Autodesk Fusion 360 part; units mm, degrees
sketch "Sketch1" plane through (0, 0, 0) normal (0, 0, 1) x (1, 0, 0)
  line L0 (0, 0) -> (53.2, 0)
  line L1 (53.2, 0) -> (53.2, 40.2)
  line L2 (53.2, 40.2) -> (0, 40.2)
  line L3 (0, 40.2) -> (0, 0)
  circle A0 centre (4.6, 4.6) radius 1.75
  circle A1 centre (4.6, 35.6) radius 1.75
  circle A2 centre (48.6, 35.6) radius 1.75
  circle A3 centre (48.6, 4.6) radius 1.75
  dimension "d1" = 53.2
  dimension "d2" = 40.2
  dimension "d3" = 4.6
  dimension "d4" = 4.6
  dimension "d5" = 4.6
  dimension "d6" = 4.6
  dimension "d7" = 4.6
  dimension "d8" = 4.6
  dimension "d9" = 4.6
  dimension "d10" = 4.6
  dimension "d11" = 3.5
  dimension "d12" = 3.5
  dimension "d13" = 3.5
  dimension "d14" = 3.5
extrude "Extrude1" add sketch "Sketch1" along normal blind 4
fillet "Fillet1" radius 4.6 4 edges at (0, 40.2, 2) (0, 0, 2) (53.2, 0, 2) (53.2, 40.2, 2)
sketch "Sketch2" plane through (0, 0, 0) normal (0, 0, -1) x (-1, 0, 0)
  arc A0 (-48.6, 40.2) -> (-53.2, 35.6) centre (-48.6, 35.6) ccw
  line L0 (-53.2, 35.6) -> (-53.2, 4.6)
  arc A1 (-53.2, 4.6) -> (-48.6, 0) centre (-48.6, 4.6) ccw
  line L1 (-48.6, 0) -> (-4.6, 0)
  arc A2 (-4.6, 0) -> (0, 4.6) centre (-4.6, 4.6) ccw
  line L2 (0, 4.6) -> (0, 35.6)
  arc A3 (0, 35.6) -> (-4.6, 40.2) centre (-4.6, 35.6) ccw
  line L3 (-4.6, 40.2) -> (-48.6, 40.2)
  circle A4 centre (-48.6, 4.6) radius 1.75
  circle A5 centre (-48.6, 35.6) radius 1.75
  circle A6 centre (-4.6, 4.6) radius 1.75
  circle A7 centre (-4.6, 35.6) radius 1.75
  line L4 (-51.6, 35.6) -> (-51.6, 4.6)
  arc A8 (-51.6, 4.6) -> (-48.6, 1.6) centre (-48.6, 4.6) ccw
  line L5 (-48.6, 1.6) -> (-4.6, 1.6)
  arc A9 (-4.6, 1.6) -> (-1.6, 4.6) centre (-4.6, 4.6) ccw
  line L6 (-1.6, 4.6) -> (-1.6, 35.6)
  arc A10 (-1.6, 35.6) -> (-4.6, 38.6) centre (-4.6, 35.6) ccw
  line L7 (-4.6, 38.6) -> (-48.6, 38.6)
  arc A11 (-48.6, 38.6) -> (-51.6, 35.6) centre (-48.6, 35.6) ccw
  dimension "d18" = 1.6
extrude "Extrude2" cut sketch "Sketch2" against normal blind 2 contours L4 A8 L5 A9 L6 A10 L7 A11
sketch "Sketch3" plane through (0, 0, 0) normal (0, 0, -1) x (-1, 0, 0)
  line L0 (-51.6, 4.6) -> (-51.6, 35.6)
  arc A0 (-48.6, 38.6) -> (-51.6, 35.6) centre (-48.6, 35.6) ccw
  line L1 (-48.6, 38.6) -> (-4.6, 38.6)
  arc A1 (-1.6, 35.6) -> (-4.6, 38.6) centre (-4.6, 35.6) ccw
  line L2 (-1.6, 35.6) -> (-1.6, 4.6)
  arc A2 (-4.6, 1.6) -> (-1.6, 4.6) centre (-4.6, 4.6) ccw
  line L3 (-4.6, 1.6) -> (-48.6, 1.6)
  arc A3 (-51.6, 4.6) -> (-48.6, 1.6) centre (-48.6, 4.6) ccw
  arc A4 (-48.6, 40.2) -> (-53.2, 35.6) centre (-48.6, 35.6) ccw
  line L4 (-53.2, 35.6) -> (-53.2, 4.6)
  arc A5 (-53.2, 4.6) -> (-48.6, 0) centre (-48.6, 4.6) ccw
  line L5 (-48.6, 0) -> (-4.6, 0)
  arc A6 (-4.6, 0) -> (0, 4.6) centre (-4.6, 4.6) ccw
  line L6 (0, 4.6) -> (0, 35.6)
  arc A7 (0, 35.6) -> (-4.6, 40.2) centre (-4.6, 35.6) ccw
  line L7 (-4.6, 40.2) -> (-48.6, 40.2)
  line L8 (0, 24.6) -> (-1.6, 24.6)
  line L9 (0, 7.6) -> (-1.6, 7.6)
  line L10 (-53.2, 28.6) -> (-51.6, 28.6)
  line L11 (-53.2, 6.6) -> (-51.6, 6.6)
  line L12 (-46.35, 40.2) -> (-46.35, 38.6)
  line L13 (-7.35, 40.2) -> (-7.35, 38.6)
  dimension "d21" = 17
  dimension "d22" = 11
  dimension "d25" = 5
  dimension "d26" = 10
  dimension "d27" = 5.75
  dimension "d73" = 39
extrude "Extrude3" cut sketch "Sketch3" against normal blind 2 contours L0 L4 L10 L11 | L2 L6 L8 L9 | L1 L7 L12 L13
sketch "Sketch4" plane through (0, 0, 2) normal (0, 0, -1) x (-1, 0, 0)
  circle A0 centre (-48.6, 4.6) radius 1.75
  circle A1 centre (-4.6, 35.6) radius 1.75
  circle A2 centre (-4.6, 4.6) radius 1.75
  circle A3 centre (-48.6, 35.6) radius 1.75
  line L0 (-53.2, 28.6) -> (-53.2, 6.6)
  line L1 (0, 7.6) -> (0, 24.6)
  line L2 (-7.35, 40.2) -> (-46.35, 40.2)
  arc A4 (-48.6, 38.6) -> (-51.6, 35.6) centre (-48.6, 35.6) ccw
  line L3 (-51.6, 35.6) -> (-51.6, 28.6)
  line L4 (-51.6, 28.6) -> (-53.2, 28.6)
  line L5 (-53.2, 6.6) -> (-51.6, 6.6)
  line L6 (-51.6, 6.6) -> (-51.6, 4.6)
  arc A5 (-51.6, 4.6) -> (-48.6, 1.6) centre (-48.6, 4.6) ccw
  line L7 (-48.6, 1.6) -> (-4.6, 1.6)
  arc A6 (-4.6, 1.6) -> (-1.6, 4.6) centre (-4.6, 4.6) ccw
  line L8 (-1.6, 4.6) -> (-1.6, 7.6)
  line L9 (-1.6, 7.6) -> (0, 7.6)
  line L10 (0, 24.6) -> (-1.6, 24.6)
  line L11 (-1.6, 24.6) -> (-1.6, 35.6)
  arc A7 (-1.6, 35.6) -> (-4.6, 38.6) centre (-4.6, 35.6) ccw
  line L12 (-4.6, 38.6) -> (-7.35, 38.6)
  line L13 (-7.35, 38.6) -> (-7.35, 40.2)
  line L14 (-46.35, 40.2) -> (-46.35, 38.6)
  line L15 (-46.35, 38.6) -> (-48.6, 38.6)
  line L16 (-51.6, 28.6) -> (-45.1, 28.6)
  line L17 (-45.1, 28.6) -> (-45.1, 6.6)
  line L18 (-45.1, 6.6) -> (-51.6, 6.6)
  line L19 (-7.35, 38.6) -> (-7.35, 31.6)
  line L20 (-7.35, 31.6) -> (-46.35, 31.6)
  line L21 (-46.35, 31.6) -> (-46.35, 38.6)
  line L22 (-1.6, 24.6) -> (-6.6, 24.6)
  line L23 (-6.6, 24.6) -> (-6.6, 7.6)
  line L24 (-6.6, 7.6) -> (-1.6, 7.6)
  line L25 (-12.1, 1.6) -> (-12.1, 8.6)
  line L26 (-12.1, 8.6) -> (-23.6, 8.6)
  line L27 (-23.6, 8.6) -> (-23.6, 1.6)
  line L28 (-25.1, 1.6) -> (-25.1, 6.1)
  line L29 (-25.1, 6.1) -> (-43.6, 6.1)
  line L30 (-43.6, 6.1) -> (-43.6, 1.6)
  dimension "d74" = 6.5
  dimension "d75" = 7
  dimension "d76" = 5
  dimension "d77" = 10.5
  dimension "d78" = 11.5
  dimension "d79" = 7
  dimension "d80" = 4.5
  dimension "d81" = 23.5
  dimension "d82" = 18.5
extrude "Extrude4" cut sketch "Sketch4" against normal blind 2 contours L0 L4 L5 L16 L17 L18 | L2 L13 L14 L19 L20 L21 | L7 L28 L29 L30 | L7 L25 L26 L27 | L1 L9 L10 L22 L23 L24
sketch "Sketch5" plane through (0, 0, 2) normal (0, 0, -1) x (-1, 0, 0)
  line L0 (-51.6, 35.6) -> (-51.6, 28.6)
  line L1 (-48.6, 1.6) -> (-43.6, 1.6)
  line L2 (-1.6, 7.6) -> (-6.6, 7.6)
  line L3 (-6.6, 24.6) -> (-1.6, 24.6)
  line L4 (-7.35, 38.6) -> (-7.35, 31.6)
  line L5 (-4.6, 38.6) -> (-7.35, 38.6)
  line L6 (-46.35, 31.6) -> (-46.35, 38.6)
  line L7 (-51.6, 28.6) -> (-45.1, 28.6)
  line L8 (-45.1, 6.6) -> (-51.6, 6.6)
  circle A0 centre (-48.6, 35.6) radius 1.75
  circle A1 centre (-4.6, 4.6) radius 1.75
  circle A2 centre (-4.6, 35.6) radius 1.75
  circle A3 centre (-48.6, 4.6) radius 1.75
  line L9 (-12.6, 8.6) -> (-6.6, 8.6)
  line L10 (-6.6, 8.6) -> (-6.6, 2.6)
  line L11 (-6.6, 2.6) -> (-12.6, 2.6)
  line L12 (-12.6, 2.6) -> (-12.6, 8.6)
  arc A4 (-4.6, 1.6) -> (-1.6, 4.6) centre (-4.6, 4.6) ccw
  line L13 (-1.6, 4.6) -> (-1.6, 7.6)
  line L14 (-1.6, 24.6) -> (-1.6, 35.6)
  arc A5 (-1.6, 35.6) -> (-4.6, 38.6) centre (-4.6, 35.6) ccw
  line L15 (-46.35, 38.6) -> (-48.6, 38.6)
  arc A6 (-48.6, 38.6) -> (-51.6, 35.6) centre (-48.6, 35.6) ccw
  line L16 (-51.6, 6.6) -> (-51.6, 4.6)
  arc A7 (-51.6, 4.6) -> (-48.6, 1.6) centre (-48.6, 4.6) ccw
  line L17 (-45.1, 28.6) -> (-45.1, 6.6)
  line L18 (-43.6, 1.6) -> (-43.6, 6.1)
  line L19 (-43.6, 6.1) -> (-25.1, 6.1)
  line L20 (-25.1, 6.1) -> (-25.1, 1.6)
  line L21 (-25.1, 1.6) -> (-23.6, 1.6)
  line L22 (-23.6, 1.6) -> (-23.6, 8.6)
  line L23 (-23.6, 8.6) -> (-12.1, 8.6)
  line L24 (-12.1, 8.6) -> (-12.1, 1.6)
  line L25 (-12.1, 1.6) -> (-4.6, 1.6)
  line L26 (-6.6, 7.6) -> (-6.6, 24.6)
  line L27 (-7.35, 31.6) -> (-46.35, 31.6)
  dimension "d49" = 6
  dimension "d51" = 6
  dimension "d83" = 1
  dimension "d84" = 5
extrude "Extrude5" cut sketch "Sketch5" against normal blind 1.3 contours L9 L10 L11 L24 L26 | L9 L11 L12 L23 L24
sketch "Sketch8" plane through (0, 0, 2) normal (0, 0, -1) x (-1, 0, 0)
  line L0 (-6.6, 24.6) -> (-1.6, 24.6)
  line L1 (-7.35, 38.6) -> (-7.35, 31.6)
  line L2 (-4.6, 38.6) -> (-7.35, 38.6)
  line L3 (-46.35, 31.6) -> (-46.35, 38.6)
  line L4 (-51.6, 28.6) -> (-45.1, 28.6)
  line L5 (-45.1, 6.6) -> (-51.6, 6.6)
  line L6 (-51.6, 35.6) -> (-51.6, 28.6)
  line L7 (-48.6, 1.6) -> (-43.6, 1.6)
  line L8 (-23.6, 8.6) -> (-6.6, 8.6)
  circle A0 centre (-48.6, 35.6) radius 1.75
  circle A1 centre (-4.6, 35.6) radius 1.75
  circle A2 centre (-48.6, 4.6) radius 1.75
  arc A3 (-1.6, 35.6) -> (-4.6, 38.6) centre (-4.6, 35.6) ccw
  line L9 (-46.35, 38.6) -> (-48.6, 38.6)
  arc A4 (-48.6, 38.6) -> (-51.6, 35.6) centre (-48.6, 35.6) ccw
  line L10 (-51.6, 6.6) -> (-51.6, 4.6)
  arc A5 (-51.6, 4.6) -> (-48.6, 1.6) centre (-48.6, 4.6) ccw
  line L11 (-6.6, 8.6) -> (-6.6, 24.6)
  line L12 (-7.35, 31.6) -> (-46.35, 31.6)
  line L13 (-45.1, 28.6) -> (-45.1, 6.6)
  line L14 (-43.6, 1.6) -> (-43.6, 6.1)
  line L15 (-43.6, 6.1) -> (-25.1, 6.1)
  line L16 (-25.1, 6.1) -> (-25.1, 1.6)
  line L17 (-25.1, 1.6) -> (-23.6, 1.6)
  line L18 (-23.6, 1.6) -> (-23.6, 8.6)
  line L19 (-1.6, 24.6) -> (-1.6, 35.6)
  line L20 (-45.1, 6.6) -> (-43.6, 6.1)
  line L21 (-7.35, 31.6) -> (-1.6, 31.6)
  line L22 (-46.35, 31.6) -> (-46.6643, 31.6)
  line L23 (-46.6643, 31.6) -> (-51.6, 31.6)
  line L24 (-6.6, 7.6) -> (-6.6, 2.6)
  line L25 (-6.6, 2.6) -> (-12.1, 2.6)
  line L26 (-12.1, 2.6) -> (-12.1, 1.6)
  line L27 (-12.1, 1.6) -> (-4.6, 1.6)
  arc A6 (-4.6, 1.6) -> (-1.6, 4.6) centre (-4.6, 4.6) ccw
  line L28 (-1.6, 4.6) -> (-1.6, 7.6)
  line L29 (-1.6, 7.6) -> (-6.6, 7.6)
  circle A7 centre (-4.6, 4.6) radius 1.75
  line L30 (-6.6, 2.6) -> (-6.6, 1.6)
extrude "Extrude8" add sketch "Sketch8" along normal blind 2 contours L1 L2 A3 L19 L21 | L3 L6 L9 A4 L22 L23 | L5 L7 L10 A5 L14 L20 | L24 L27 A6 L28 L29 L30
sketch "Sketch9" plane through (0, 0, 2) normal (0, 0, -1) x (-1, 0, 0)
  line L0 (-45.1, 6.6) -> (-43.6, 6.1)
  line L1 (-43.6, 6.1) -> (-25.1, 6.1)
  line L2 (-25.1, 6.1) -> (-25.1, 1.6)
  line L3 (-25.1, 1.6) -> (-23.6, 1.6)
  line L4 (-23.6, 1.6) -> (-23.6, 8.6)
  line L5 (-23.6, 8.6) -> (-6.6, 8.6)
  line L6 (-6.6, 8.6) -> (-6.6, 24.6)
  line L7 (-6.6, 24.6) -> (-1.6, 24.6)
  line L8 (-1.6, 24.6) -> (-1.6, 31.6)
  line L9 (-1.6, 31.6) -> (-7.35, 31.6)
  line L10 (-7.35, 31.6) -> (-46.35, 31.6)
  line L11 (-46.35, 31.6) -> (-51.6, 31.6)
  line L12 (-51.6, 31.6) -> (-51.6, 28.6)
  line L13 (-51.6, 28.6) -> (-45.1, 28.6)
  line L14 (-45.1, 28.6) -> (-45.1, 6.6)
  line L15 (-7.6, 10.6) -> (-9.6, 10.6)
  line L16 (-9.6, 10.6) -> (-9.6, 13.6)
  line L17 (-9.6, 13.6) -> (-7.6, 13.6)
  line L18 (-7.6, 13.6) -> (-7.6, 10.6)
  dimension "d85" = 2
  dimension "d86" = 1
  dimension "d87" = 3
  dimension "d88" = 2
extrude "Extrude9" cut sketch "Sketch9" against normal blind 1.5 contours L15 L16 L17 L18
sketch "Sketch10" plane through (0, 0, 2) normal (0, 0, -1) x (-1, 0, 0)
  line L0 (-9.6, 10.6) -> (-9.6, 13.6)
  line L1 (-9.6, 13.6) -> (-7.6, 13.6)
  line L2 (-7.6, 13.6) -> (-7.6, 10.6)
  line L3 (-7.6, 10.6) -> (-9.6, 10.6)
  line L4 (-45.1, 6.6) -> (-43.6, 6.1)
  line L5 (-43.6, 6.1) -> (-25.1, 6.1)
  line L6 (-25.1, 6.1) -> (-25.1, 1.6)
  line L7 (-25.1, 1.6) -> (-23.6, 1.6)
  line L8 (-23.6, 1.6) -> (-23.6, 8.6)
  line L9 (-23.6, 8.6) -> (-6.6, 8.6)
  line L10 (-6.6, 8.6) -> (-6.6, 24.6)
  line L11 (-6.6, 24.6) -> (-1.6, 24.6)
  line L12 (-1.6, 24.6) -> (-1.6, 31.6)
  line L13 (-1.6, 31.6) -> (-7.35, 31.6)
  line L14 (-7.35, 31.6) -> (-46.35, 31.6)
  line L15 (-46.35, 31.6) -> (-51.6, 31.6)
  line L16 (-51.6, 31.6) -> (-51.6, 28.6)
  line L17 (-51.6, 28.6) -> (-45.1, 28.6)
  line L18 (-45.1, 28.6) -> (-45.1, 6.6)
  line L19 (-43.6, 7.4) -> (-40.6, 7.4)
  line L20 (-40.6, 7.4) -> (-40.6, 13.4)
  line L21 (-40.6, 13.4) -> (-43.6, 13.4)
  line L22 (-43.6, 13.4) -> (-43.6, 7.4)
  line L23 (-6.6, 1.6) -> (-43.6, 1.6)
  dimension "d91" = 6
  dimension "d92" = 3
  dimension "d93" = 8
  dimension "d94" = 5.8
extrude "Extrude10" cut sketch "Sketch10" against normal blind 2 contours L19 L20 L21 L22
equation "d1 = 50 mm + ( ( 2 * 1.6 ) * 1 mm )"
equation "d2 = 37 mm + ( ( 2 * 1.6 ) * 1 mm )"
equation "d3 = 3 mm + 1.6 mm"
equation "d4 = d3"
equation "d5 = d4"
equation "d6 = d3"
equation "d7 = d3"
equation "d8 = d7"
equation "d9 = d4"
equation "d10 = d5"
equation "d17 = 3 mm + 1.6 mm"
CAD build for the part. Positions are in the model's coordinates, mm. A direction names the side the tool comes from. Round coordinates to 2 decimals unless told otherwise and drop trailing zeros. Order: outer loops, then holes, each group sorted by start corner. A loop starts at its lowest first (then second) coordinate and runs counter-clockwise, first axis right, second up. Notation, with made-up numbers: (10.5, 32) -> (19.5, 32) arc R35 cw to (19.5, 64) -> close; hole circle Ø10 at (65, 31). An arc over 180 degrees is marked (long way). Write item = value, one per line. Start each with the question number.
(1) Cut at C-C, the plane x = 27. List the corners of the cut face in (y, z), then the cut area to 3 significant figures.
(2) Cut at A-A, the plane x = 42. List the corners of the cut face in (y, z), then the cut area to 3 significant figures.
(3) Which spindle directions (+Z, -Z, +X, -X, +Y, -Y) get a long thin tool onto all of the face, cutting with end or side? Do faces 4 (the flat face through (46.35, 36, 2)), 5 (the flat face through (3, 7.6, 2)), 6 (the flat face through (7.6, 12, 3)). Say none if no direction does.
(4) Cut at B-B, the plane z = 1.4. State how many separate pieces and enclosed holes the cut face has, then the cut area to 3 significant figures.
(5) Probe line 1 (X direction, y = 4.6, z = 1.25); line 2 (X direction, y = 4.6, z = 2.6); line 3 (X direction, y = 4.6, z = 3.6). List the from-to ranges inside material, lowest first. Write a range as [from, to].
(6) Cut at D-D, the plane y = 26.5. List the corners of the cut face in (x, z), then the cut area to 3 significant figures.
(7) Pull direction X, two halves, no side cores. Call faces 1 (the flat face through (25.1, 4, 3)), 2 (the flat face through (0, 30, 2)), 3 (the flat face through (6, 40.2, 2)): released by +X, released by -X, zero draft, split by the parting line, or undercut.
(8) Pin check, flat tips, straight feed: P1, Ø0.6, axis at x = 10, z = 2.5, coming from the +Y side; P2, Ø2, axis at y = 11.5, z = 3, coming from the +X side; P3, Ø0.6, axis at y = 26.5, z = 1, coming from the +X side. Stop position of each tip, or through.
Model answer:
q1.outline = (0, 0) -> (1.6, 0) -> (1.6, 4) -> (0, 4) -> close; (6.1, 2) -> (31.6, 2) -> (31.6, 4) -> (6.1, 4) -> close
q1.area = 57.4 mm2
q2.outline = (0, 0) -> (1.6, 0) -> (1.6, 4) -> (0, 4) -> close; (6.1, 2) -> (7.4, 2) -> (7.4, 4) -> (6.1, 4) -> close; (13.4, 2) -> (31.6, 2) -> (31.6, 4) -> (13.4, 4) -> close
q2.area = 45.4 mm2
q3.face_4 = +Z, -Z, +Y
q3.face_5 = +Z, -Z, -X
q3.face_6 = -Z
q4.separate_pieces = 3
q4.enclosed_holes = 4
q4.area = 254 mm2
q5.line_1 = [0, 2.85], [6.35, 6.6], [43.6, 46.85], [50.35, 53.2]
q5.line_2 = [0, 2.85], [6.35, 6.6], [23.6, 25.1], [43.6, 46.85], [50.35, 53.2]
q5.line_3 = [0, 2.85], [6.35, 12.1], [23.6, 25.1], [43.6, 46.85], [50.35, 53.2]
q6.outline = (0, 0) -> (1.6, 0) -> (1.6, 2) -> (45.1, 2) -> (45.1, 4) -> (0, 4) -> close
q6.area = 93.4 mm2
q7.face_1 = undercut
q7.face_2 = released by -X
q7.face_3 = zero draft
q8.P1 = 31.6
q8.P2 = 45.1
q8.P3 = 1.6
